Design review of the part built by this model. Coordinates are the model's own, in mm. A direction names the side the tool comes from. Give positions to 0.01 mm unless a question says otherwise; leave off trailing zeros. Order: outer loops, then holes, each group sorted by start corner. A loop starts at its lowest first (then second) coordinate and runs counter-clockwise, first axis right, second up.
```python
from build123d import *

# Parameters (mm, degrees)
SKETCH4_R           = 16.6
SKETCH4_R_2         = 6.15
BOSS_EXTRUDE1_DEPTH = 12
BOSS_EXTRUDE2_DEPTH = 1.5
SKETCH6_R           = 1.2
CUT_EXTRUDE1_DEPTH  = 27.365128484
SKETCH7_R           = 1.5
CUT_EXTRUDE2_DEPTH  = 28.08080501
FILLET1_R           = 1
FILLET2_R           = 1
SKETCH8_W           = 20
SKETCH8_H           = 5
CUT_EXTRUDE3_DEPTH  = 1.5


with BuildPart() as part:
    # Sketch4 → Boss-Extrude1 (new body)
    with BuildSketch(Plane(origin=(0, 0, 0), x_dir=(1, 0, 0), z_dir=(0, 1, 0))):
        with Locations(Location((0, 0, 0), (0, 0, 270))):
            Circle(SKETCH4_R)
        with Locations(Location((0, 0, 0), (0, 0, 270))):
            Circle(SKETCH4_R_2, mode=Mode.SUBTRACT)
    extrude(amount=-BOSS_EXTRUDE1_DEPTH)

    # Sketch5 → Boss-Extrude2 (add)
    with BuildSketch(Plane.XZ.offset(12)):
        with BuildLine():
            Line((11.2, 10.859097568), (11.2, -7.7))
            Line((11.2, -7.7), (-11.2, -7.7))
            Line((-11.2, -7.7), (-11.2, 10.859097568))
            ThreePointArc((-11.2, 10.859097568), (0, -15.6), (11.2, 10.859097568))
        make_face()
    extrude(amount=BOSS_EXTRUDE2_DEPTH)

    # Sketch6 → Cut-Extrude1 (cut, through all)
    with BuildSketch(Plane.XZ.offset(12)):
        with Locations((9, -5.5)):
            Circle(SKETCH6_R)
        with Locations((9, 5.5)):
            Circle(SKETCH6_R)
        with Locations((-9, 5.5)):
            Circle(SKETCH6_R)
        with Locations((-9, -5.5)):
            Circle(SKETCH6_R)
    extrude(amount=-CUT_EXTRUDE1_DEPTH, mode=Mode.SUBTRACT)

    # Sketch7 → Cut-Extrude2 (cut, through all)
    with BuildSketch(Plane(origin=(0, 0, 0), x_dir=(1, 0, 0), z_dir=(0, 1, 0))):
        with Locations(Location((0, 12.6, 0), (0, 0, 270))):
            Circle(SKETCH7_R)
        with Locations(Location((12.6, 0, 0), (0, 0, 270))):
            Circle(SKETCH7_R)
        with Locations(Location((-12.6, 0, 0), (0, 0, 270))):
            Circle(SKETCH7_R)
        with Locations(Location((0, -12.6, 0), (0, 0, 270))):
            Circle(SKETCH7_R)
    extrude(amount=-CUT_EXTRUDE2_DEPTH, mode=Mode.SUBTRACT)

    # Fillet1
    fillet1_edges = [part.edges().sort_by_distance(p)[0] for p in [
        (-11.2, -12.75, 10.859097568),
        (11.2, -12.75, 10.859097568),
    ]]
    fillet(fillet1_edges, radius=FILLET1_R)

    # Fillet2
    # the kernel refuses this fillet: 1 mm, written as the material it takes off along each edge
    with BuildSketch(Plane(origin=(0, -13.5, 0), x_dir=(-0.7369271930502395, 0, 0.675972123791429), z_dir=(0.675972123791429, 0, 0.7369271930502395))) as fillet2_piece_1:
        with BuildLine():
            CenterArc((15.6 - FILLET2_R, -FILLET2_R), FILLET2_R, 0, 90)
            Line((15.6 - FILLET2_R, 0), (15.6, 0))
            Line((15.6, 0), (15.6, -FILLET2_R))
        make_face()
    revolve(axis=Axis((0, -13.5, 0), (0, -1, 0)), revolution_arc=265.059373538, mode=Mode.SUBTRACT)

    # Sketch8 → Cut-Extrude3 (cut)
    with BuildSketch(Plane.XZ.offset(12)):
        with Locations((0, 16.2)):
            Rectangle(SKETCH8_W, SKETCH8_H)
        Polygon((3.35, 11.5), (-5.2, 11.5), (-5.2, 9), (-3.65, 9), (-3.65, 4.5), (3.35, 4.5), align=None)
    extrude(amount=-CUT_EXTRUDE3_DEPTH, mode=Mode.SUBTRACT)


solid = part.part
```
1. Take a section at C-C (z = 12.6). State the section outline as (x, y) points, then the cut area to 3 significant figures.
Recorded:
outline: (-10.81, -12) - (-1.5, -12) - (-1.5, 0) - (-10.81, 0) - close; (1.5, -12) - (10.81, -12) - (10.81, 0) - (1.5, 0) - close
area: 223 mm2
2. Draft analysis for pull direction X (two halves, no side actions). For faces 4 (the face through (5, -11, 13.7)), 5 (the face through (12, -13, 9)), 6 (the face through (0.73, -5.916, -16.584)), 7 (the face through (-5.2, -11, 10)), state which applies: pulls with the +X half, pulls with the -X half, needs draft (parallel to the pull), parting line crosses it, or undercut.
Recorded:
face 4: needs draft
face 5: undercut
face 6: parting line crosses it
face 7: undercut
3. Take a section at B-B (y = -5.25). State how many separate pieces and enclosed holes the cut face has, then the cut area to 3 significant figures.
Recorded:
separate pieces: 1
enclosed holes: 9
area: 701 mm2
4. Take a section at A-A (x = 0). State the section outline as (y, z) points, then the cut area to 3 significant figures.
Recorded:
outline: (-13.5, -14.6) arc R1 ccw to (-12.5, -15.6) - (-12, -15.6) - (-12, -16.6) - (0, -16.6) - (0, -14.1) - (-13.5, -14.1) - close; (-13.5, -11.1) - (0, -11.1) - (0, -6.15) - (-12, -6.15) - (-12, -7.7) - (-13.5, -7.7) - close; (-10.5, 6.15) - (0, 6.15) - (0, 11.1) - (-10.5, 11.1) - close; (-10.5, 14.1) - (0, 14.1) - (0, 16.6) - (-10.5, 16.6) - close
area: 175 mm2
5. Machinability: for faces 1 (the face through (-3, -11, 11.5)), 2 (the face through (0, -13, -7.7)), 3 (the face through (-13.93, -6.66, 0.69)), which of the approach directions +Z, -Z, +X, -X, +Y, -Y give a long, thin tool a straight path to every point of the face, cutting with its end or side? Answer none if there is none.
Recorded:
face 1: -Y
face 2: +Z, -Y
face 3: +Y, -Y
6. For pin 1 (6 mm diameter, centred on y = -3, z = -11, fed in from -X); pin 2 (0.8 mm diameter, centred on y = -12.5, z = -3.5, fed in from +X); pin 3 (0.8 mm diameter, centred on x = 1.5, y = -11.5, fed in from -Z), all flat-tipped, find the tip position at first contact; note any pin that passes through.
Recorded:
pin 1: stops at x = -14.55
pin 2: stops at x = 15.29
pin 3: stops at z = -16.56
7. For line 1 along X through (y, z) = (-5, 0); line 2 along X through (y, z) = (-2, 1); line 3 along Y through (x, z) = (-7, 15), list the stretches that pass through material, from the lowest coordinate up.
Recorded:
line 1: x = -16.6 to -14.1, -11.1 to -6.15, 6.15 to 11.1, 14.1 to 16.6
line 2: x = -16.57 to -13.72, -11.48 to -6.07, 6.07 to 11.48, 13.72 to 16.57
line 3: y = -10.5 to 0
